Geometry check sheet. Reference: the model listing, model coordinates, mm. A direction names the side the tool comes from. Give positions to 0.01 mm unless a question says otherwise; leave off trailing zeros. Loops run counter-clockwise (first coordinate to the right, second up) from the corner with the lowest first, then second, coordinate; pieces in that order, holes last. Notation, with made-up numbers: (0.5, 57) -> (25.5, 57) arc R27 cw to (25.5, 73) -> close; hole circle Ø9 at (80, 13.5). An arc over 180 degrees is marked (long way). Answer as a JSON object with one key per item and string values.
Autodesk Inventor part; units mm, degrees
ref_plane "YZ Plane" through (0, 0, 0) normal (1, 0, 0) x (0, 1, 0)
ref_plane "XZ Plane" through (0, 0, 0) normal (0, 1, 0) x (-1, 0, 0)
ref_plane "XY Plane" through (0, 0, 0) normal (0, 0, 1) x (1, 0, 0)
sketch "Skizze1" plane through (0, 0, 0) normal (0, 1, 0) x (-1, 0, 0)
  circle A0 centre (0, 0) radius 3
  circle A1 centre (0, 0) radius 16
  dimension "d0" = 6
  dimension "d1" = 32
extrude "Extrusion1" add sketch "Skizze1" along normal blind 0.7
sketch "Skizze2" plane through (0, 0.7, 0) normal (0, 1, 0) x (1, 0, 0)
  circle A0 centre (0, 0) radius 16
  line L0 (-15.9511, -1.25) -> (-12, -1.25)
  arc A1 (-12, -1.25) -> (-12, 1.25) centre (-12, 0) ccw
  line L1 (-12, 1.25) -> (-15.9511, 1.25)
  point P0 (-13.9755, -1.25)
  dimension "d4" = 12
  dimension "d5" = 2.5
extrude "Extrusion2" cut sketch "Skizze2" against normal blind 0.7 contours L1 A1 L0 A0 picked at (-13.3315, -0.139)
pattern_circular "Runde Anordnung1" count 8 over 360 about axis through (0, -10, 0) along (0, 1, 0) of "Extrusion2"
properties part number "Disc"
1) Section check A-A on z = 0. Record the cut outline in (x, y), plus the area to 4 significant figures.
Geometry check:
{"outline": "(-10.75, 0) -> (-3, 0) -> (-3, 0.7) -> (-10.75, 0.7) -> close; (3, 0) -> (10.75, 0) -> (10.75, 0.7) -> (3, 0.7) -> close", "area": "10.85 mm2"}
2) Depth check by flat-ended pin: P1, Ø3.5, axis at x = 0, z = 0, coming from the -Y side. Enter the tip coordinate at first touch or a pass-through.
Geometry check:
{"P1": "passes through"}
3) Tool access check on faces 1 (the face through (10.75, 0.35, -8.98)), 2 (the face through (-6.188, 0.345, -14.755)). Record the directions out of +Z, -Z, +X, -X, +Y, -Y that give a thin tool (end or side, any length) a straight path to the whole face; none if there is none.
Geometry check:
{"face 1": "+Y, -Y", "face 2": "-Z, -X, +Y, -Y"}
4) Section check D-D on x = -5. Record the cut outline in (y, z), plus the area to 3 significant figures.
Geometry check:
{"outline": "(0, -15.2) -> (0.7, -15.2) -> (0.7, 15.2) -> (0, 15.2) -> close", "area": "21.3 mm2"}
5) Material ranges on line 1 along Z through (x, y) = (0, 0.45); line 2 along X through (y, z) = (0.3, -8); line 3 along X through (y, z) = (0.4, -10), recorded low to high. Write a range as from..to.
Geometry check:
{"line 1": "z = -10.75..-3, 3..10.75", "line 2": "x = -13.86..-9.77, -7.33..7.33, 9.77..13.86", "line 3": "x = -12.49..-11.77, -8.23..8.23, 11.77..12.49"}
6) Draft check along X on faces 3 (the face through (6.06, 0.35, -14.81)), 4 (the face through (0.2, 0.7, -3.3)), 5 (the face through (7.6, 0.4, -7.6)). Enter one of: pulls with the +X half, pulls with the -X half, needs draft (parallel to the pull), parting line crosses it, or undercut.
Geometry check:
{"face 3": "pulls with the +X half", "face 4": "needs draft", "face 5": "undercut"}
7) Section check C-C on z = -8.5. Record the cut outline in (x, y), plus the area to 3 significant figures.
Geometry check:
{"outline": "(-13.56, 0) -> (-10.27, 0) -> (-10.27, 0.7) -> (-13.56, 0.7) -> close; (-7.24, 0) -> (7.24, 0) -> (7.24, 0.7) -> (-7.24, 0.7) -> close; (10.27, 0) -> (13.56, 0) -> (13.56, 0.7) -> (10.27, 0.7) -> close", "area": "14.7 mm2"}
